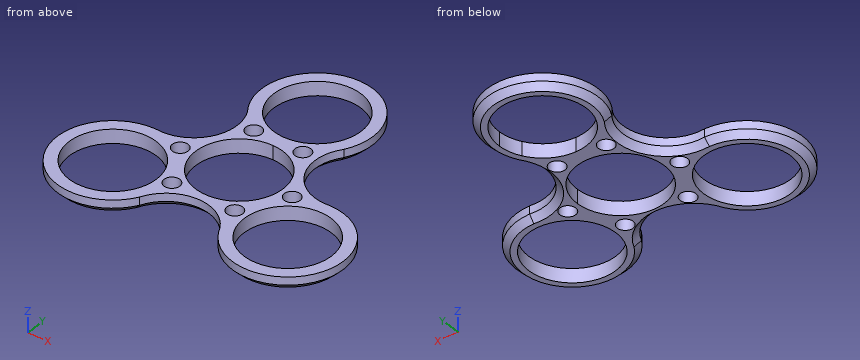
```python
from build123d import *

# Parameters (mm, degrees)
F0_R       = 11
F0_R_2     = 2
F1_DEPTH   = 3.5
F2_C1_SIZE = 1.5
F2_C2_SIZE = 1.5
F2_C3_SIZE = 1.5
F2_C4_SIZE = 1.5
F2_C5_SIZE = 1.5
F2_C6_SIZE = 1.5


with BuildPart() as f1:
    # F0 (on Top) → F1 (new body)
    with BuildSketch(Plane.XY):
        with BuildLine():
            ThreePointArc((22.164837833, 1.2031249106), (11.390396953, 6.576248747), (12.124355653, 18.5937501788))
            ThreePointArc((12.124355653, 18.5937501788), (0, 39.5937501788), (-12.124355653, 18.5937501788))
            ThreePointArc((-12.124355653, 18.5937501788), (-11.390396953, 6.576248747), (-22.164837833, 1.2031249106))
            ThreePointArc((-22.164837833, 1.2031249106), (-34.2891934859, -19.7968750894), (-10.04048218, -19.7968750894))
            ThreePointArc((-10.04048218, -19.7968750894), (0, -13.152497494), (10.04048218, -19.7968750894))
            ThreePointArc((10.04048218, -19.7968750894), (34.2891934859, -19.7968750894), (22.164837833, 1.2031249106))
        make_face()
        with Locations((-22.164837833, -12.7968750894)):
            Circle(F0_R, mode=Mode.SUBTRACT)
        with Locations((-7.9711980778, -11.7872301109)):
            Circle(F0_R_2, mode=Mode.SUBTRACT)
        with Locations((-14.1936397552, -1.0096449785)):
            Circle(F0_R_2, mode=Mode.SUBTRACT)
        with Locations((7.9711980778, -11.7872301109)):
            Circle(F0_R_2, mode=Mode.SUBTRACT)
        with Locations((22.164837833, -12.7968750894)):
            Circle(F0_R, mode=Mode.SUBTRACT)
        with BuildLine():
            ThreePointArc((0, 11), (7.7781745931, 7.7781745931), (11, 0))
            ThreePointArc((11, 0), (-7.7781745931, -7.7781745931), (0, 11))
        make_face(mode=Mode.SUBTRACT)
        with Locations((14.1936397552, -1.0096449785)):
            Circle(F0_R_2, mode=Mode.SUBTRACT)
        with Locations((-6.2224416774, 12.7968750894)):
            Circle(F0_R_2, mode=Mode.SUBTRACT)
        with Locations((6.2224416774, 12.7968750894)):
            Circle(F0_R_2, mode=Mode.SUBTRACT)
        with BuildLine():
            ThreePointArc((9.5262794416, 20.0937501788), (5.5, 16.0674707372), (0, 14.5937501788))
            ThreePointArc((0, 14.5937501788), (-5.5, 16.0674707372), (-9.5262794416, 20.0937501788))
            ThreePointArc((-9.5262794416, 20.0937501788), (-2.8470094961, 36.218934268), (11, 25.5937501788))
            ThreePointArc((11, 25.5937501788), (10.6251840892, 22.7467406827), (9.5262794416, 20.0937501788))
        make_face(mode=Mode.SUBTRACT)
    extrude(amount=F1_DEPTH)

    # F2: chamfer of 1.5 on 6 edges, made by hand

    # F2_c1
    f2_c1_edges = [f1.edges().sort_by_distance(p)[0] for p in [
        (0, -13.152497494, 0),
    ]]
    chamfer(f2_c1_edges, length=F2_C1_SIZE)

    # F2_c2
    f2_c2_edges = [f1.edges().sort_by_distance(p)[0] for p in [
        (-11.390396953, 6.576248747, 0),
    ]]
    chamfer(f2_c2_edges, length=F2_C2_SIZE)

    # F2_c3
    f2_c3_edges = [f1.edges().sort_by_distance(p)[0] for p in [
        (11.390396953, 6.576248747, 0),
    ]]
    chamfer(f2_c3_edges, length=F2_C3_SIZE)

    # F2_c4
    f2_c4_edges = [f1.edges().sort_by_distance(p)[0] for p in [
        (34.2891934859, -19.7968750894, 0),
    ]]
    chamfer(f2_c4_edges, length=F2_C4_SIZE)

    # F2_c5
    f2_c5_edges = [f1.edges().sort_by_distance(p)[0] for p in [
        (-34.2891934859, -19.7968750894, 0),
    ]]
    chamfer(f2_c5_edges, length=F2_C5_SIZE)

    # F2_c6
    f2_c6_edges = [f1.edges().sort_by_distance(p)[0] for p in [
        (0, 39.5937501788, 0),
    ]]
    chamfer(f2_c6_edges, length=F2_C6_SIZE)


solid = f1.part
```
Work out the finished part from the listing and answer in its coordinate system (mm). Coordinates: 2 decimals unless noted, no trailing zeros. Use a Markdown table: item, result.
Item 1: Consider probe 1 along X at (y, z) = (-22, 2.1); probe 2 along Y at (x, z) = (-1.5, 1.8); probe 3 along X at (y, z) = (-21, 2.15). Determine where each line is inside the solid, lowest interval first. Write a range as from..to.
Evaluation:
| item | result |
|---|---|
| probe 1 | x = -32.71..-28.19, -16.14..-11.61, 11.61..16.14, 28.19..32.71 |
| probe 2 | y = -13.26..-10.9, 10.9..14.7, 36.49..39.51 |
| probe 3 | x = -33.51..-29.49, -14.84..-10.82, 10.82..14.84, 29.49..33.51 |
Item 2: Find section A-A, the plane z = 2.4. State how many separate pieces and enclosed holes the cut face has, and give its area (3 significant figures).
Evaluation:
| item | result |
|---|---|
| separate pieces | 1 |
| enclosed holes | 10 |
| area | 874 mm2 |
Item 3: Given pin 1 Ø1.5 at (y, z) = (10.5, 3) entering from +X; pin 2 Ø1.5 at (x, y) = (-13, 6.5) entering from -Z; pin 3 Ø1.5 at (x, z) = (-20, 1) entering from -Y, each flat-ended and moving along its own axis, determine where each tip first touches the part or whether it passes through.
Evaluation:
| item | result |
|---|---|
| pin 1 | stops at x = 10.17 |
| pin 2 | passes through |
| pin 3 | stops at y = -26.7 |
